Study the drawing (mm; zero at the part's minimum x, y, z) and answer. Round coordinates to 2 decimals unless told otherwise and drop trailing zeros. Order: outer loops, then holes, each group sorted by start corner. A loop starts at its lowest first (then second) coordinate and runs counter-clockwise, first axis right, second up. Notation, with made-up numbers: (-7.75, 86) -> (40.25, 86) arc R23 cw to (40.25, 96) -> close; hole circle Ø2 at (49, 67.25). An arc over 180 degrees is marked (long way). Use one line per item in the form item = value.
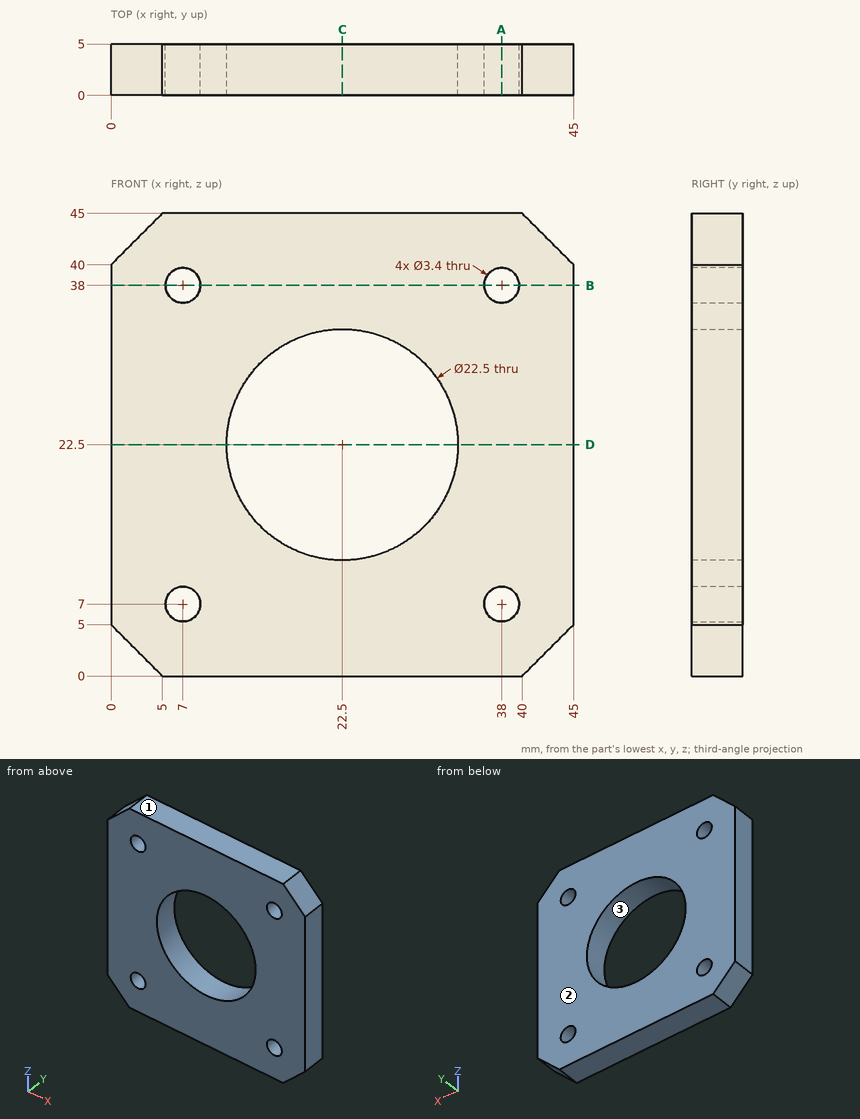
Item 1: Determine the mould class of the marked faces 1, 2 and 3 for opening direction Z: released by +Z, released by -Z, zero draft, split by the parting line, or undercut.
Findings:
face_1 = released by +Z
face_2 = zero draft
face_3 = undercut
Item 2: Consider line 1 along X through (y, z) = (3.15, 38); line 2 along Z through (x, y) = (22.5, 2.2). Determine where each line is inside the solid, lowest interval first.
Findings:
line_1 = 0 to 5.3, 8.7 to 36.3, 39.7 to 45
line_2 = 0 to 11.25, 33.75 to 45
Item 3: The part is cut by section D-D, the plane z = 22.5. Give the vertices of the cut face in (x, y), and give its area (4 significant figures).
Findings:
outline = (0, 0) -> (11.25, 0) -> (11.25, 5) -> (0, 5) -> close; (33.75, 0) -> (45, 0) -> (45, 5) -> (33.75, 5) -> close
area = 112.5 mm^2
Item 4: The part is cut by section C-C, the plane x = 22.5. Give the vertices of the cut face in (y, z), and give its area (4 significant figures).
Findings:
outline = (0, 0) -> (5, 0) -> (5, 11.25) -> (0, 11.25) -> close; (0, 33.75) -> (5, 33.75) -> (5, 45) -> (0, 45) -> close
area = 112.5 mm^2
Item 5: The part is cut by section B-B, the plane z = 38. Give the vertices of the cut face in (x, y), and give its area (3 significant figures).
Findings:
outline = (0, 0) -> (5.3, 0) -> (5.3, 5) -> (0, 5) -> close; (8.7, 0) -> (36.3, 0) -> (36.3, 5) -> (8.7, 5) -> close; (39.7, 0) -> (45, 0) -> (45, 5) -> (39.7, 5) -> close
area = 191 mm^2
Item 6: The part is cut by section A-A, the plane x = 38. Give the vertices of the cut face in (y, z).
Findings:
outline = (0, 0) -> (5, 0) -> (5, 5.3) -> (0, 5.3) -> close; (0, 8.7) -> (5, 8.7) -> (5, 36.3) -> (0, 36.3) -> close; (0, 39.7) -> (5, 39.7) -> (5, 45) -> (0, 45) -> close
